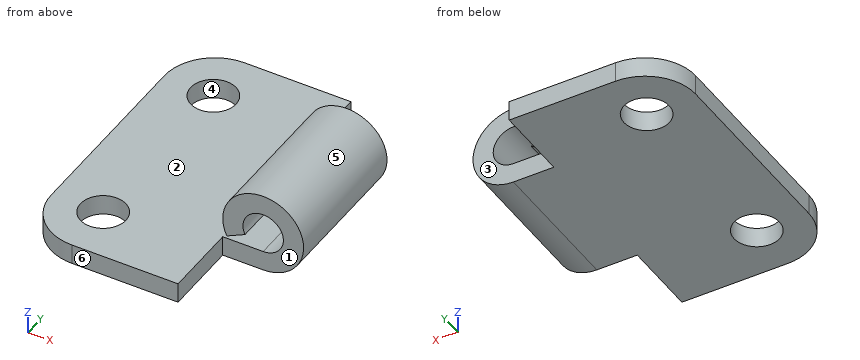
from build123d import *

# Parameters (mm, degrees)
BASE_FLANGE1_DEPTH = 4
HEM2_START         = -14
HEM2_DEPTH         = 28
SKETCH12_R         = 4.5
CUT_EXTRUDE1_DEPTH = 10
FILLET1_R          = 10


# Read off the part's stored shape, not the designer's step: Hem2
# Sheet-metal steps are written as plain solids
with BuildPart() as part:
    # Sketch1 → Base-Flange1 (new body)
    with BuildSketch(Plane.XY):
        Polygon((15.5, 14), (23.5, 14), (23.5, -14), (15.5, -14), (15.5, -29), (-15.5, -29), (-15.5, 29), (15.5, 29), align=None)
    extrude(amount=-BASE_FLANGE1_DEPTH)

    # Hem2 outline → Hem2 (add)
    with BuildSketch(Plane(origin=(0, 0, 0), x_dir=(1, 0, 0), z_dir=(0, 1, 0)).offset(HEM2_START)):
        with BuildLine():
            Line((19.904823815, -2.246515413), (16.30964763, -0.493030826))
            ThreePointArc((16.30964763, -0.493030826), (27.739354115, -10.784384769), (23.5, 4))
            Line((23.5, 4), (23.5, 0))
            ThreePointArc((23.5, 0), (25.619677058, -7.392192385), (19.904823815, -2.246515413))
        make_face()
    extrude(amount=HEM2_DEPTH)

    # Sketch12 → Cut-Extrude1 (cut)
    with BuildSketch(Plane.XY):
        with Locations((-5.5, 18.5)):
            Circle(SKETCH12_R)
        with Locations((-5.5, -18.5)):
            Circle(SKETCH12_R)
    extrude(amount=-CUT_EXTRUDE1_DEPTH, mode=Mode.SUBTRACT)

    # Fillet1
    fillet1_edges = [part.edges().sort_by_distance(p)[0] for p in [
        (-15.5, -29, -2),
        (-15.5, 29, -2),
    ]]
    fillet(fillet1_edges, radius=FILLET1_R)


solid = part.part
Source: CAD feature listing. Evaluate the final solid. Frame: model axes, mm. Face numbers are marked on the shaded views. A direction names the side the tool comes from. Coordinates: 2 decimals unless noted, no trailing zeros. Loops run counter-clockwise (first coordinate to the right, second up) from the corner with the lowest first, then second, coordinate; pieces in that order, holes last. Notation, with made-up numbers: (-14.75, -26.5) -> (-9.75, -26.5) arc R35 cw to (-9.75, 6.5) -> close; hole circle Ø3 at (23, 51). An arc over 180 degrees is marked (long way). Answer in a Markdown table with one row per item. Add a question column.
Q1. Section C-C on y = 0. Return the cut outline in (x, z).
Q2. Section B-B on x = -2.5. Return the cut outline in (y, z).
Q3. Ray query, line 1 along Y through (x, z) = (-5.5, -3.1); line 2 along X through (y, z) = (1.75, 4); line 3 along Z through (x, y) = (-13, -23.5). Return the intervals inside material, ascending.
Q4. Section A-A on z = 4. Return the cut outline in (x, y).
Q5. Pull-direction query (Y, two-part tool) for the marked faces 4, 5 and 6; classes: pulls with the +Y half, pulls with the -Y half, needs draft (parallel to the pull), parting line crosses it, or undercut.
Q6. Contact query for flat-ended pins moving along their axis: pin 1 Ø9 at (x, z) = (23.5, 4) entering from -Y; pin 2 Ø7 at (x, y) = (-5.5, -18.5) entering from -Z; pin 3 Ø8 at (x, z) = (26, 8) entering from +Y; pin 4 Ø3 at (y, z) = (-20, -1.5) entering from +X. Output: stop coordinate, or through.
Q7. Section D-D on z = 7.25. Return the cut outline in (x, y).
Q8. Reachability of the marked faces 1, 2 and 3 from +Z, -Z, +X, -X, +Y, -Y: full face, straight path, thin tool, end or side. Return the list, or none.
Computed values:
| question | item | result |
|---|---|---|
| 1 | outline | (-15.5, -4) -> (23.5, -4) arc R8 ccw (long way) to (16.31, 0.49) -> (19.9, 2.25) arc R4 cw (long way) to (23.5, 0) -> (-15.5, 0) -> close |
| 2 | outline | (-29, -4) -> (-21.85, -4) -> (-21.85, 0) -> (-29, 0) -> close; (-15.15, -4) -> (15.15, -4) -> (15.15, 0) -> (-15.15, 0) -> close; (21.85, -4) -> (29, -4) -> (29, 0) -> (21.85, 0) -> close |
| 3 | line 1 | y = -29 to -23, -14 to 14, 23 to 29 |
| 3 | line 2 | x = 15.5 to 19.5, 27.5 to 31.5 |
| 3 | line 3 | z = -4 to 0 |
| 4 | outline | (15.5, -14) -> (19.5, -14) -> (19.5, 14) -> (15.5, 14) -> close; (27.5, -14) -> (31.5, -14) -> (31.5, 14) -> (27.5, 14) -> close |
| 5 | face 4 | undercut |
| 5 | face 5 | needs draft |
| 5 | face 6 | pulls with the -Y half |
| 6 | pin 1 | stops at y = -14 |
| 6 | pin 2 | passes through |
| 6 | pin 3 | stops at y = 14 |
| 6 | pin 4 | stops at x = 15.5 |
| 7 | outline | (16.19, -14) -> (21.17, -14) -> (21.17, 14) -> (16.19, 14) -> close; (25.83, -14) -> (30.81, -14) -> (30.81, 14) -> (25.83, 14) -> close |
| 8 | face 1 | +Z, -Z, +X, -Y |
| 8 | face 2 | -X, +Y, -Y |
| 8 | face 3 | +Z, -Z, +X, +Y |
